Can you work these out from the model? Positions are in its coordinate system, mm. A direction names the side the tool comes from. Round coordinates to 2 decimals unless told otherwise and drop trailing zeros. Write item = value, one per line. Start each with the question number.
1) Thinking about a two-plate mould opening in X: for faces 4 (the face through (18, 4, 3.7)), 5 (the face through (5.43, 5.8, -17.2)), 6 (the face through (14, 1, -5.2)), which applies, +X half, -X half, draft (parallel to the pull), parting line (faces both ways), or undercut?
2) I'm going to push flat-ended pins straight in: pin 1 (1 mm diameter, centred on x = -0.5, z = 8.5, fed in from -Y); pin 2 (4 mm diameter, centred on x = -8, z = 13.86, fed in from -Y); pin 3 (2.5 mm diameter, centred on x = -17.5, z = 2, fed in from +Y); pin 4 (1.5 mm diameter, centred on x = -10, y = 5.5, fed in from -Z). Where does each tip first touch, or does it pass through?
3) Imagine slicing it at A-A, the plane x = 0. State how many separate pieces and enclosed holes the cut face has, then the cut area to 3 significant figures.
4) For faces 1 (the face through (16.293, 1.282, 9.38)), 2 (the face through (6.221, 4.022, -10.612)), 3 (the face through (-12.01, 4.02, -13.4)), which set-ups out of +Z, -Z, +X, -X, +Y, -Y let a thin tool reach every point of the face, with its end or its side?
5) If I drill on line 1 (X direction, y = 0.5, z = 9); line 2 (Z direction, x = 1.5, y = 2.5); line 3 (X direction, y = 4.5, z = 11.5), over which ranges is the centre line in solid material (lowest first)?
from build123d import *

# Parameters (mm, degrees)
CUT_EXTRUDE1_DEPTH           = 3.6
M4_CLEARANCE_HOLE1_D         = 4.5
CUT_EXTRUDE2_DEPTH           = 2.6
M3_CLEARANCE_HOLE2_D         = 3.4
FILLET1_R                    = 0.4
CHAMFER1_SIZE                = 1
CIRPATTERN1_COUNT            = 6
FILLET1_OF_CIRPATTERN1_R     = 0.4
CHAMFER1_OF_CIRPATTERN1_SIZE = 1
CHAMFER2_SIZE                = 0.4


with BuildPart() as part:
    # Sketch1 → Revolve1 (revolve)
    with BuildSketch(Plane.XY, mode=Mode.PRIVATE) as revolve1_sk:
        Polygon((8.1, 0), (20.1, 0), (20.1, 6), (7.7, 6), (7.7, 5.2), (8.1, 4.8), align=None)
    revolve(revolve1_sk.sketch.rotate(Axis((0, 16.469304641, 0), (0, -1, 0)), 180), axis=Axis((0, 16.469304641, 0), (0, -1, 0)))

    # Sketch2 → Cut-Extrude1 (cut)
    with BuildSketch(Plane(origin=(0, 6, 0), x_dir=(1, 0, 0), z_dir=(0, 1, 0))):
        with BuildLine():
            Line((16, 3.7), (19.756517912, 3.7))
            ThreePointArc((19.756517912, 3.7), (20.1, 0), (19.756517912, -3.7))
            Line((19.756517912, -3.7), (16, -3.7))
            ThreePointArc((16, -3.7), (12.3, 0), (16, 3.7))
        make_face()
    cut_extrude1 = extrude(amount=-CUT_EXTRUDE1_DEPTH, mode=Mode.SUBTRACT)

    # M4 Clearance Hole1 (through all)
    with Locations(Plane(origin=(0, 2.4, 0), x_dir=(1, 0, 0), z_dir=(0, 1, 0))):
        with Locations((16, 0)):
            m4_clearance_hole1 = Hole(M4_CLEARANCE_HOLE1_D / 2)

    # Sketch8 → Cut-Extrude2 (cut)
    with BuildSketch(Plane.XZ):
        Polygon((3.233161507, -16), (1.616580754, -13.2), (-1.616580754, -13.2), (-3.233161507, -16), (-1.616580754, -18.8), (1.616580754, -18.8), align=None)
    cut_extrude2 = extrude(amount=-CUT_EXTRUDE2_DEPTH, mode=Mode.SUBTRACT)

    # M3 Clearance Hole2 (through all)
    with Locations(Plane(origin=(0, 2.6, 0), x_dir=(-1, 0, 0), z_dir=(0, -1, 0))):
        with Locations((0, 16)):
            m3_clearance_hole2 = Hole(M3_CLEARANCE_HOLE2_D / 2)

    # Fillet1
    fillet1_edges = [part.edges().sort_by_distance(p)[0] for p in [
        (19.756517912, 4.2, -3.7),
        (19.756517912, 4.2, 3.7),
    ]]
    fillet(fillet1_edges, radius=FILLET1_R)

    # Chamfer1
    chamfer1_edges = [part.edges().sort_by_distance(p)[0] for p in [
        (-1.7, 2.6, -16),
    ]]
    chamfer(chamfer1_edges, length=CHAMFER1_SIZE)

    # CirPattern1: Cut-Extrude1, M4 Clearance Hole1, Cut-Extrude2, M3 Clearance Hole2 ×6 about axis
    cirpattern1_axis = Axis((0, 0, 0), (0, 1, 0))
    add([cut_extrude1.rotate(cirpattern1_axis, i * 360 / CIRPATTERN1_COUNT) for i in range(1, CIRPATTERN1_COUNT)], mode=Mode.SUBTRACT)
    add([m4_clearance_hole1.rotate(cirpattern1_axis, i * 360 / CIRPATTERN1_COUNT) for i in range(1, CIRPATTERN1_COUNT)], mode=Mode.SUBTRACT)
    add([cut_extrude2.rotate(cirpattern1_axis, i * 360 / CIRPATTERN1_COUNT) for i in range(1, CIRPATTERN1_COUNT)], mode=Mode.SUBTRACT)
    add([m3_clearance_hole2.rotate(cirpattern1_axis, i * 360 / CIRPATTERN1_COUNT) for i in range(1, CIRPATTERN1_COUNT)], mode=Mode.SUBTRACT)

    # Fillet1 of CirPattern1
    fillet1_of_cirpattern1_edges = [part.edges().sort_by_distance(p)[0] for p in [
        (6.673964962, 4.2, -18.959646402),
        (13.08255295, 4.2, -15.259646402),
        (-13.08255295, 4.2, -15.259646402),
        (-6.673964962, 4.2, -18.959646402),
        (-19.756517912, 4.2, 3.7),
        (-19.756517912, 4.2, -3.7),
        (-6.673964962, 4.2, 18.959646402),
        (-13.08255295, 4.2, 15.259646402),
        (13.08255295, 4.2, 15.259646402),
        (6.673964962, 4.2, 18.959646402),
    ]]
    fillet(fillet1_of_cirpattern1_edges, radius=FILLET1_OF_CIRPATTERN1_R)

    # Chamfer1 of CirPattern1
    chamfer1_of_cirpattern1_edges = [part.edges().sort_by_distance(p)[0] for p in [
        (-14.706406461, 2.6, -6.527756814),
        (-13.006406461, 2.6, 9.472243186),
        (1.7, 2.6, 16),
        (14.706406461, 2.6, 6.527756814),
        (13.006406461, 2.6, -9.472243186),
    ]]
    chamfer(chamfer1_of_cirpattern1_edges, length=CHAMFER1_OF_CIRPATTERN1_SIZE)

    # Chamfer2
    chamfer2_edges = [part.edges().sort_by_distance(p)[0] for p in [
        (6.15, 6, 10.652112467),
        (5.612862844, 6, 17.121763621),
        (-6.15, 6, 10.652112467),
        (-12.021450832, 6, 13.421763621),
        (-12.3, 6, 0),
        (-17.634313676, 6, -3.7),
        (-6.15, 6, -10.652112467),
        (-5.612862844, 6, -17.121763621),
        (6.15, 6, -10.652112467),
        (12.021450832, 6, -13.421763621),
        (12.3, 6, 0),
        (17.634313676, 6, 3.7),
        (5.612862844, 6, -17.121763621),
        (0, 6, -20.1),
        (13.122486484, 6, -15.032202838),
        (6.45702629, 6, -18.880508075),
        (-12.021450832, 6, -13.421763621),
        (-17.407110616, 6, -10.05),
        (-6.45702629, 6, -18.880508075),
        (-13.122486484, 6, -15.032202838),
        (-17.634313676, 6, 3.7),
        (-17.407110616, 6, 10.05),
        (-19.579512774, 6, -3.848305237),
        (-19.579512774, 6, 3.848305237),
        (-5.612862844, 6, 17.121763621),
        (0, 6, 20.1),
        (-13.122486484, 6, 15.032202838),
        (-6.45702629, 6, 18.880508075),
        (12.021450832, 6, 13.421763621),
        (17.407110616, 6, 10.05),
        (6.45702629, 6, 18.880508075),
        (13.122486484, 6, 15.032202838),
        (17.634313676, 6, -3.7),
        (17.407110616, 6, -10.05),
        (19.579512774, 6, 3.848305237),
        (19.579512774, 6, -3.848305237),
    ]]
    chamfer(chamfer2_edges, length=CHAMFER2_SIZE - 0.0001)  # a hair under: the kernel refuses the full size


solid = part.part
Reported:
q1.face_4 = draft
q1.face_5 = +X half
q1.face_6 = undercut
q2.pin_1 = 0
q2.pin_2 = through
q2.pin_3 = 2.4
q2.pin_4 = -11.38
q3.separate_pieces = 4
q3.enclosed_holes = 0
q3.area = 90.4 mm²
q4.face_1 = -Y
q4.face_2 = +Y
q4.face_3 = -Z, +Y
q5.line_1 = -17.97 to -16.51, -11.2 to 11.2, 16.51 to 17.97
q5.line_2 = -20.04 to -18.8, -13.2 to -7.96, 7.96 to 13.2, 18.8 to 20.04
q5.line_3 = -16.49 to -10.85, -5.15 to 5.15, 10.85 to 16.49
